Autodesk Inventor part; units mm, degrees
ref_plane "YZ Plane" through (0, 0, 0) normal (1, 0, 0) x (0, 1, 0)
ref_plane "XZ Plane" through (0, 0, 0) normal (0, 1, 0) x (-1, 0, 0)
ref_plane "XY Plane" through (0, 0, 0) normal (0, 0, 1) x (1, 0, 0)
sketch "PCB" plane through (0, 0, 0) normal (0, 1, 0) x (-1, 0, 0)
  line L0 (0, 0) -> (60, 0)
  line L1 (60, 0) -> (60, -98)
  line L2 (60, -98) -> (0, -98)
  line L3 (0, -98) -> (0, 0)
  dimension "d0" = 98
  dimension "d1" = 60
extrude "PCB_Extr" add sketch "PCB" along normal blind 1.6
sketch "Mounting" plane through (0, 1.6, 0) normal (0, 1, 0) x (1, 0, 0)
  circle A0 centre (-57.5, 2.5) radius 1.25
  circle A1 centre (-57.5, 95.5) radius 1.25
  circle A2 centre (-2.5, 95.5) radius 1.25
  circle A3 centre (-2.5, 2.5) radius 1.25
  line L0 (-60, 0) -> (0, 0)
  line L1 (-60, 98) -> (-60, 0)
  line L2 (0, 98) -> (-60, 98)
  line L3 (0, 0) -> (0, 98)
  dimension "d4" = 2.5
  dimension "d5" = 2.5
  dimension "d6" = 2.5
  dimension "d7" = 2.5
  dimension "d8" = 2.5
  dimension "d9" = 2.5
  dimension "d10" = 2.5
  dimension "d11" = 2.5
  dimension "d12" = 2.5
  dimension "d13" = 2.5
  dimension "d14" = 2.5
  dimension "d15" = 2.5
extrude "Mounting_Extr" cut sketch "Mounting" against normal through all contours A0 | A1 | A2 | A3
sketch "Pinning" plane through (0, 1.6, 0) normal (0, 1, 0) x (1, 0, 0)
  circle A0 centre (-57.5, 10) radius 0.5
  circle A1 centre (-57.5, 12.54) radius 0.5
  circle A2 centre (-57.5, 15.08) radius 0.5
  circle A3 centre (-57.5, 25.24) radius 0.5
  circle A4 centre (-57.5, 20.16) radius 0.5
  circle A5 centre (-57.5, 27.78) radius 0.5
  circle A6 centre (-57.5, 22.7) radius 0.5
  circle A7 centre (-57.5, 17.62) radius 0.5
  line L0 (-60, 0) -> (0, 0)
  line L1 (-60, 98) -> (-60, 0)
  line L2 (-59.0965, 29.05) -> (-55.5485, 29.05)
  circle A8 centre (-57.5, 48.1) radius 0.5
  circle A9 centre (-57.5, 45.56) radius 0.5
  circle A10 centre (-57.5, 43.02) radius 0.5
  circle A11 centre (-57.5, 32.86) radius 0.5
  circle A12 centre (-57.5, 37.94) radius 0.5
  circle A13 centre (-57.5, 30.32) radius 0.5
  circle A14 centre (-57.5, 35.4) radius 0.5
  circle A15 centre (-57.5, 40.48) radius 0.5
  dimension "d18" = 1
  dimension "d19" = 1
  dimension "d20" = 1
  dimension "d21" = 1
  dimension "d22" = 1
  dimension "d23" = 1
  dimension "d24" = 1
  dimension "d25" = 1
  dimension "d26" = 10
  dimension "d27" = 2.5
  dimension "d28" = 2.54
  dimension "d29" = 2.54
  dimension "d30" = 2.54
  dimension "d31" = 2.54
  dimension "d32" = 2.54
  dimension "d33" = 2.54
  dimension "d34" = 2.54
  dimension "d38" = 1.27
extrude "Pinning_Extr" cut sketch "Pinning" against normal through all
equation "\"d5\" = d4"
equation "\"d6\" = d4"
equation "\"d7\" = d4"
equation "\"d9\" = d8"
equation "\"d10\" = d8"
equation "\"d11\" = d8"
equation "\"d12\" = d8"
equation "\"d13\" = d8"
equation "\"d14\" = d8"
equation "\"d15\" = d8"
equation "\"d19\" = d18"
equation "\"d20\" = d18"
equation "\"d21\" = d18"
equation "\"d22\" = d18"
equation "\"d23\" = d18"
equation "\"d24\" = d18"
equation "\"d25\" = d18"
equation "\"d29\" = d28"
equation "\"d30\" = d28"
equation "\"d31\" = d28"
equation "\"d32\" = d28"
equation "\"d33\" = d28"
equation "\"d34\" = d28"
properties part number "Mounting_PCB"
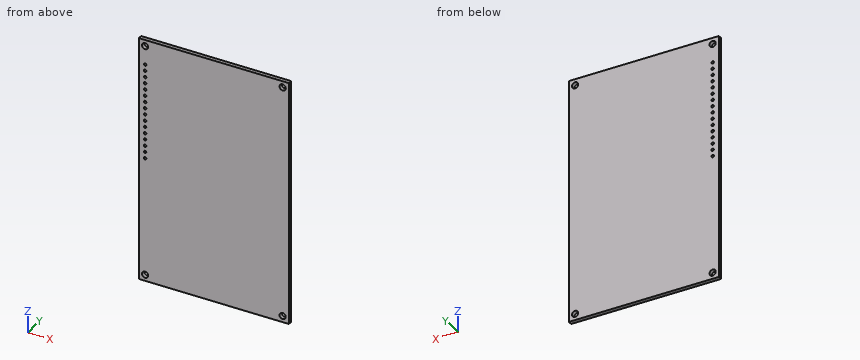
The model under review builds one solid part; all positions refer to its coordinate system, in mm. Round coordinates to 2 decimals unless told otherwise and drop trailing zeros. Order: outer loops, then holes, each group sorted by start corner. A loop starts at its lowest first (then second) coordinate and runs counter-clockwise, first axis right, second up. Notation, with made-up numbers: (-1, 49) -> (22, 49) arc R26 cw to (22, 76) -> close; hole circle Ø2 at (37.5, 73.25). An arc over 180 degrees is marked (long way). One line per item, written item: value. Start each with the question number.
Q1. Clearance check with a flat-ended pin moving along its axis: pin 1 Ø12 at (x, z) = (-33.5, -58) entering from -Y. State where the tip first meets the part, or that it passes through.
Q2. Wall thickness on line 1 (X direction, y = 0.4, z = -95.5); line 2 (X direction, y = 0.5, z = -15); line 3 (X direction, y = 0.4, z = -25.5): over which ranges is each line inside the solid? List them lowest first.
Q3. Take a section at A-A (z = -2.5). Write out the cut boundary in (x, y), and give its area (3 significant figures).
Q4. Take a section at B-B (x = -2.5). Write out the cut boundary in (y, z).
Reported:
1. pin 1: stops at y = 0
2. line 1: x = -60 to -58.75, -56.25 to -3.75, -1.25 to 0
2. line 2: x = -60 to -57.99, -57.01 to 0
2. line 3: x = -60 to -57.93, -57.07 to 0
3. outline: (-60, 0) -> (-58.75, 0) -> (-58.75, 1.6) -> (-60, 1.6) -> close; (-56.25, 0) -> (-3.75, 0) -> (-3.75, 1.6) -> (-56.25, 1.6) -> close; (-1.25, 0) -> (0, 0) -> (0, 1.6) -> (-1.25, 1.6) -> close
3. area: 88.0 mm2
4. outline: (0, -98) -> (1.6, -98) -> (1.6, -96.75) -> (0, -96.75) -> close; (0, -94.25) -> (1.6, -94.25) -> (1.6, -3.75) -> (0, -3.75) -> close; (0, -1.25) -> (1.6, -1.25) -> (1.6, 0) -> (0, 0) -> close
